Here's how the part is built. I have some questions about the finished solid (model axes, mm). Face numbers are marked on the shaded views. Round coordinates to 2 decimals unless told otherwise and drop trailing zeros. Write each loop counter-clockwise with the first axis right and the second up, starting at its lowest first coordinate (ties: lowest second). Pieces come first, ordered by that corner, then holes. Notation, with made-up numbers: (24, -7.5) -> (52, -7.5) arc R36 ccw to (52, 28.5) -> close; hole circle Ø8 at (23.5, 20). An arc over 180 degrees is marked (long way). Answer in a Markdown table with one row per item.
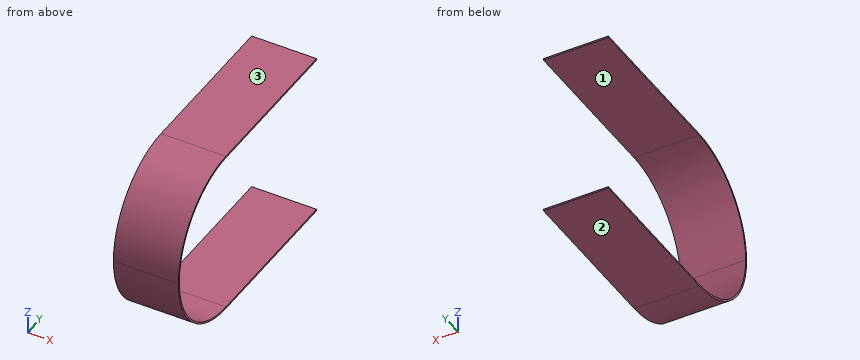
from build123d import *

# Parameters (mm, degrees)
F4_DEPTH = 20


# Not quite as in the source:
# - a feature of the source that left no trace in its solid (it failed there, or was rolled back) is left out


with BuildPart() as f4:
    # F2 (on Right) → F4 (new body)
    with BuildSketch(Plane.YZ):
        with BuildLine():
            ThreePointArc((-25.25, 0), (-17.854446225, 17.854446225), (0, 25.25))
            Line((0, 25.25), (49.0651577711, 25.25))
            Line((49.0651577711, 25.25), (49.0651577711, 25.75))
            Line((49.0651577711, 25.75), (0, 25.75))
            ThreePointArc((0, 25.75), (-18.2079996156, 18.2079996156), (-25.75, 0))
            Line((-25.75, 0), (-25.25, 0))
        make_face()
        with BuildLine():
            ThreePointArc((0, -25.25), (-17.854446225, -17.854446225), (-25.25, 0))
            Line((-25.25, 0), (-25.75, 0))
            ThreePointArc((-25.75, 0), (-18.2079996156, -18.2079996156), (0, -25.75))
            Line((0, -25.75), (49.0651577711, -25.75))
            Line((49.0651577711, -25.75), (49.0651577711, -25.25))
            Line((49.0651577711, -25.25), (0, -25.25))
        make_face()
    extrude(amount=F4_DEPTH)


solid = f4.part
1) I want a section at A-A, the plane y = 8. List the corners of the cut face in (x, z) for me.
Response:
| item | result |
|---|---|
| outline | (0, -25.75) -> (20, -25.75) -> (20, -25.25) -> (0, -25.25) -> close; (0, 25.25) -> (20, 25.25) -> (20, 25.75) -> (0, 25.75) -> close |
2) We'd pull the mould along Z, two halves only. Please class the marked faces 1, 2 and 3: +Z half, -Z half, draft (parallel to the pull), parting line (faces both ways), or undercut.
Response:
| item | result |
|---|---|
| face 1 | undercut |
| face 2 | -Z half |
| face 3 | +Z half |
3) I need wall thicknesses on line 1 (Z direction, x = 11, y = 13); line 2 (Z direction, x = 15.5, y = -21); line 3 (Y direction, x = 9, z = -5.5). Which ranges of each line are inside material? Lowest first, please. Write a range as [from, to].
Response:
| item | result |
|---|---|
| line 1 | z = [-25.75, -25.25], [25.25, 25.75] |
| line 2 | z = [-14.9, -14.02], [14.02, 14.9] |
| line 3 | y = [-25.16, -24.64] |
4) I want a section at C-C, the plane y = -15.5. List the corners of the cut face in (x, z) for me, and give its area (3 significant figures).
Response:
| item | result |
|---|---|
| outline | (0, -20.56) -> (20, -20.56) -> (20, -19.93) -> (0, -19.93) -> close; (0, 19.93) -> (20, 19.93) -> (20, 20.56) -> (0, 20.56) -> close |
| area | 25.2 mm^2 |
5) I want a section at D-D, the plane z = 12.5. List the corners of the cut face in (x, y) for me.
Response:
| item | result |
|---|---|
| outline | (0, -22.51) -> (20, -22.51) -> (20, -21.94) -> (0, -21.94) -> close |
6) For pin 1 (5 mm diameter, centred on x = 3.5, z = -4.5, fed in from +Y); pin 2 (2 mm diameter, centred on x = 6.5, z = 3, fed in from +Y); pin 3 (3 mm diameter, centred on x = 11, z = 8.5, fed in from -Y); pin 4 (8 mm diameter, centred on x = 14, y = -2, fed in from -Z), each with a flat end and sliding along its axis, tell me the tip position at first contact or that it passes through.
Response:
| item | result |
|---|---|
| pin 1 | stops at y = -24.26 |
| pin 2 | stops at y = -24.93 |
| pin 3 | stops at y = -24.78 |
| pin 4 | stops at z = -25.75 |
7) I want a section at B-B, the plane x = 8.5. List the corners of the cut face in (y, z) for me.
Response:
| item | result |
|---|---|
| outline | (0, -25.75) -> (49.07, -25.75) -> (49.07, -25.25) -> (0, -25.25) arc R25.25 cw to (0, 25.25) -> (49.07, 25.25) -> (49.07, 25.75) -> (0, 25.75) arc R25.75 ccw to start |
